```python
from build123d import *

# Parameters (mm, degrees)
SKETCH1_R         = 7.9375
EXTRUDE1_DEPTH    = 6.9453125
SKETCH7_OUTSIDE_W = 121.588
SKETCH7_OUTSIDE_H = 125.272
SKETCH7_OUTSIDE_R = 11.90625
EXTRUDE2_DEPTH    = 25.4
EXTRUDE2_TAPER    = 60


with BuildPart() as part:
    # Sketch1 → Extrude1 (new body, symmetric)
    with BuildSketch(Plane.XY):
        Polygon((-11.90625, 6.874076643), (-11.90625, -6.874076643), (0, -13.748153285), (11.90625, -6.874076643), (11.90625, 6.874076643), (0, 13.748153285), align=None)
        Circle(SKETCH1_R, mode=Mode.SUBTRACT)
    extrude(amount=EXTRUDE1_DEPTH, both=True)

    # Sketch7 outside → Extrude2 (cut)
    with BuildSketch(Plane.XY.offset(6.9453125)):
        Rectangle(SKETCH7_OUTSIDE_W, SKETCH7_OUTSIDE_H)
        Circle(SKETCH7_OUTSIDE_R, mode=Mode.SUBTRACT)
    extrude(amount=-EXTRUDE2_DEPTH, taper=EXTRUDE2_TAPER, mode=Mode.SUBTRACT)


solid = part.part
```
Here's how the part is built. I have some questions about the finished solid (model axes, mm). Round coordinates to 2 decimals unless told otherwise and drop trailing zeros. Order: outer loops, then holes, each group sorted by start corner. A loop starts at its lowest first (then second) coordinate and runs counter-clockwise, first axis right, second up. Notation, with made-up numbers: M 40.25,55 L 44.25,55 A33 ccw 44.25,91 Z; hole C 43.5,49 d5. An arc over 180 degrees is marked long. Answer as CSV lines item,"result".
Item 1: Please list where these lines run through material, in increasing order: L1, parallel to X at y = -0.25, z = 4.5; L2, parallel to Y at x = -7, z = -3.5; L3, parallel to Y at x = -0.5, z = 5.75. Write a range as [from, to].
From the geometry:
L1,"[-11.91, -7.93], [7.93, 11.91]"
L2,"[-9.71, -3.74], [3.74, 9.71]"
L3,"[-13.46, -7.92], [7.92, 13.46]"
Item 2: We'd pull the mould along X, two halves only. Please class faces 1 (the conical face through (10.71, -6.15, 6.69)), 2 (the flat face through (2, -8, 6.945)), 3 (the conical face through (-10.68, -6.2, 6.69)), 4 (the cylindrical face through (-1.72, -7.75, -0.1)): +X half, -X half, draft (parallel to the pull), parting line (faces both ways), or undercut.
From the geometry:
face 1,"+X half"
face 2,"draft"
face 3,"-X half"
face 4,"undercut"
Item 3: For pin 1 (4 mm diameter, centred on x = -6, z = 1, fed in from -Y), with a flat end and sliding along its axis, tell me the tip position at first contact or that it passes through.
From the geometry:
pin 1,"y = -11.44"
Item 4: Imagine slicing it at A-A on z = -5.5. List the corners of the cut face in (x, y) for me (1 decimal).
From the geometry:
outline,"M -11.9,-6.9 L 0,-13.7 L 11.9,-6.9 L 11.9,6.9 L 0,13.7 L -11.9,6.9 Z; hole C 0,0 d15.9"
